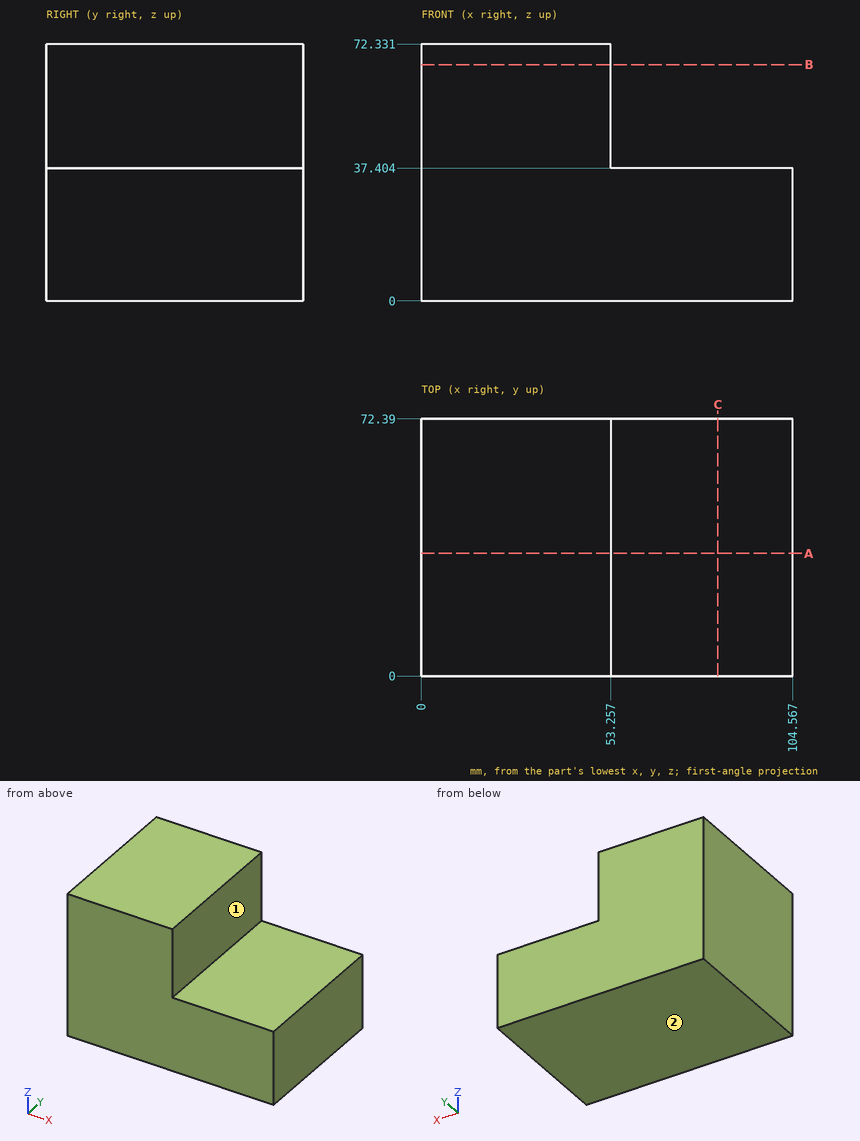
Design review of the part shown in the three views and the two pictorial views. Dimensions are in mm from the part's minimum x, y and z. A direction names the side the tool comes from. Give positions to 0.01 mm unless a question says otherwise; leave off trailing zeros. Loops run counter-clockwise (first coordinate to the right, second up) from the corner with the lowest first, then second, coordinate; pieces in that order, holes last. Notation, with made-up numbers: M -37,-27.75 L 21,-27.75 A25 cw 21,-14.75 Z; hole C -3,47 d4. An arc over 180 degrees is marked long. Put each result on its own line as item: value. Start each with the question number.
(1) Add section B-B, the plane z = 66.5. Write out the cut boundary in (x, y).
(2) Wall thickness on L1, parallel to Z at x = 87.5, y = 38; L2, parallel to X at y = 39, z = 46: over which ranges is each line inside the solid? List them lowest first.
(3) For pin 1 (15.5 mm diameter, centred on x = 80, y = 40, fed in from +Z), flat-tipped, find the tip position at first contact; note if it passes through.
(4) Add section A-A, the plane y = 34.5. Write out the cut boundary in (x, z).
(5) Machinability: for the marked faces 1 and 2, which of the approach directions +Z, -Z, +X, -X, +Y, -Y give a long, thin tool a straight path to every point of the face, cutting with its end or side? Answer none if there is none.
(6) Add section C-C, the plane x = 83.5. Write out the cut boundary in (y, z), then the cut area to 3 significant figures.
Result:
1. outline: M 0,0 L 53.26,0 L 53.26,72.39 L 0,72.39 Z
2. L1: z = 0 to 37.4
2. L2: x = 0 to 53.26
3. pin 1: stops at z = 37.4
4. outline: M 0,0 L 104.57,0 L 104.57,37.4 L 53.26,37.4 L 53.26,72.33 L 0,72.33 Z
5. face 1: +Z, +X, +Y, -Y
5. face 2: -Z, +X, -X, +Y, -Y
6. outline: M 0,0 L 72.39,0 L 72.39,37.4 L 0,37.4 Z
6. area: 2,710 mm^2
